Can you work these out from the model? Positions are in its coordinate system, mm. Face numbers are marked on the shaded views. A direction names the side the tool comes from. Coordinates: 2 decimals unless noted, no trailing zeros. Write each loop counter-clockwise with the first axis right and the second up, starting at its lowest first coordinate (ties: lowest second). Pieces come first, ordered by that corner, then holes. Notation, with made-up numbers: (71, 87) - (106, 87) arc R8 cw to (106, 100) - close; hole circle Ø9 at (6, -12.5). An arc over 180 degrees is marked (long way). Write each question's results on one line, items separated by ' | '. Start each with the question number.
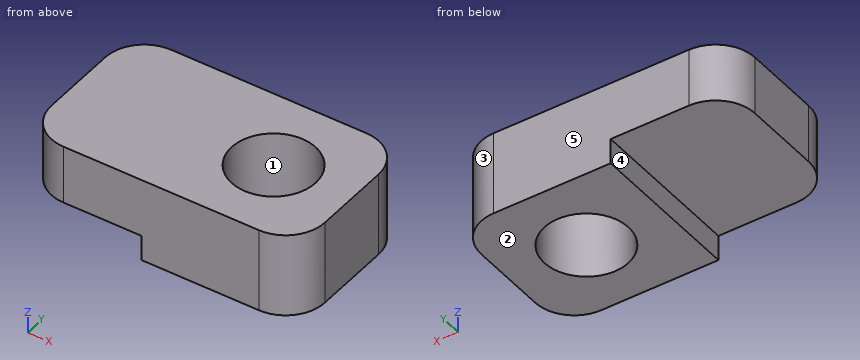
```python
from build123d import *

# Parameters (mm, degrees)
F2_DEPTH = 8
F3_R     = 2.15
F4_DEPTH = 4.3
F5_R     = 2


# Not quite as in the source:
# - a feature names something its author has since deleted; it is built from what else it names


with BuildPart() as f2:
    # F1 (on Front) → F2 (new body)
    with BuildSketch(Plane.XZ):
        Polygon((6, -3), (6, -4.3), (14, -4.3), (14, 0), (0, 0), (0, -3), align=None)
    extrude(amount=F2_DEPTH)

    # F3 (on face) → F4 (cut, through all)
    with BuildSketch(Plane.XY):
        with Locations((10, -4)):
            Circle(F3_R)
    extrude(amount=-F4_DEPTH, mode=Mode.SUBTRACT)

    # F5
    f5_edges = [f2.edges().sort_by_distance(p)[0] for p in [
        (14, -8, -2.15),
        (14, 0, -2.15),
        (0, -8, -1.5),
        (0, 0, -1.5),
    ]]
    fillet(f5_edges, radius=F5_R)


solid = f2.part
```
Q1. If we section it at B-B (y = -4): Please give me the cut outline in (x, z).
Q2. I need wall thicknesses on line 1 along Y through (x, z) = (10, -2.35); line 2 along Z through (x, y) = (1.25, -4.25); line 3 along X through (y, z) = (-4.5, -1.75). Which ranges of each line are inside material? Lowest first, please. Write a range as from..to.
Q3. If we section it at C-C (z = -3.7): Please give me the cut outline in (x, y).
Q4. If we section it at A-A (x = 10): Please give me the cut outline in (y, z).
Q5. Thinking about a two-plate mould opening in Y: for the marked faces 1, 2 and 3, which applies, pulls with the +Y half, pulls with the -Y half, needs draft (parallel to the pull), parting line crosses it, or undercut?
Q6. For the marked faces 4 and 5, which set-ups out of +Z, -Z, +X, -X, +Y, -Y let a thin tool reach every point of the face, with its end or its side?
Q7. If we section it at D-D (z = -2.8): Please give me the cut outline in (x, y).
Q8. I'm going to push flat-ended pins straight in: pin 1 Ø2.5 at (x, y) = (10, -4) entering from +Z; pin 2 Ø2 at (x, y) = (7.5, -7) entering from +Z; pin 3 Ø0.6 at (y, z) = (-3.5, -3.5) entering from -X. Where does each tip first touch, or does it pass through?
Answer list:
1) outline: (0, -3) - (6, -3) - (6, -4.3) - (7.85, -4.3) - (7.85, 0) - (0, 0) - close; (12.15, -4.3) - (14, -4.3) - (14, 0) - (12.15, 0) - close
2) line 1: y = -8..-6.15, -1.85..0 | line 2: z = -3..0 | line 3: x = 0..7.91, 12.09..14
3) outline: (6, -8) - (12, -8) arc R2 ccw to (14, -6) - (14, -2) arc R2 ccw to (12, 0) - (6, 0) - close; hole circle Ø4.3 at (10, -4)
4) outline: (-8, -4.3) - (-6.15, -4.3) - (-6.15, 0) - (-8, 0) - close; (-1.85, -4.3) - (0, -4.3) - (0, 0) - (-1.85, 0) - close
5) face 1: undercut | face 2: needs draft | face 3: pulls with the +Y half
6) face 4: -Z, -X, +Y, -Y | face 5: +Z, -Z, +X, -X, +Y
7) outline: (0, -6) arc R2 ccw to (2, -8) - (12, -8) arc R2 ccw to (14, -6) - (14, -2) arc R2 ccw to (12, 0) - (2, 0) arc R2 ccw to (0, -2) - close; hole circle Ø4.3 at (10, -4)
8) pin 1: passes through | pin 2: stops at z = 0 | pin 3: stops at x = 6
